Autodesk Inventor part; units mm, degrees
ref_plane "YZ Plane" through (0, 0, 0) normal (1, 0, 0) x (0, 1, 0)
ref_plane "XZ Plane" through (0, 0, 0) normal (0, 1, 0) x (-1, 0, 0)
ref_plane "XY Plane" through (0, 0, 0) normal (0, 0, 1) x (1, 0, 0)
sketch "Sketch1" plane through (0, 0, 0) normal (0, 1, 0) x (-1, 0, 0)
  line L0 (-9.5, 12.5) -> (9.5, 12.5)
  line L1 (12.5, 9.5) -> (12.5, -9.5)
  line L2 (9.5, -12.5) -> (-9.5, -12.5)
  line L3 (-12.5, -9.5) -> (-12.5, 9.5)
  line L4 (-12.5, 12.5) -> (12.5, -12.5) construction
  line L5 (12.5, 12.5) -> (-12.5, -12.5) construction
  line L6 (-10, -10) -> (10, -10) construction
  line L7 (10, -10) -> (10, 10) construction
  line L8 (10, 10) -> (-10, 10) construction
  line L9 (-10, 10) -> (-10, -10) construction
  line L10 (-10, -10) -> (10, 10) construction
  line L11 (10, -10) -> (-10, 10) construction
  circle A0 centre (10, 10) radius 1.2
  circle A1 centre (10, -10) radius 1.2
  circle A2 centre (-10, 10) radius 1.2
  circle A3 centre (-10, -10) radius 1.2
  arc A4 (12.5, 9.5) -> (9.5, 12.5) centre (9.5, 9.5) ccw
  arc A5 (9.5, -12.5) -> (12.5, -9.5) centre (9.5, -9.5) ccw
  arc A6 (-9.5, 12.5) -> (-12.5, 9.5) centre (-9.5, 9.5) ccw
  arc A7 (-12.5, -9.5) -> (-9.5, -12.5) centre (-9.5, -9.5) ccw
  point P0 (0, 0)
  dimension "d0" = 25
  dimension "d1" = 25
  dimension "d2" = 20
  dimension "d3" = 20
  dimension "d4" = 2.4
  dimension "d7" = 20
  dimension "d10" = 20
  dimension "d13" = 3
extrude "Extrusion1" add sketch "Sketch1" along normal blind 3
sketch "Sketch2" plane through (0, 3, 0) normal (0, 1, 0) x (1, 0, 0)
  line L0 (4, -4) -> (-4, -4)
  line L1 (-4, -4) -> (-4, 4)
  line L2 (-4, 4) -> (4, 4)
  line L3 (4, 4) -> (4, -4)
  line L4 (4, -4) -> (-4, 4) construction
  line L5 (-4, -4) -> (4, 4) construction
  point P0 (0, 0)
  dimension "d16" = 8
  dimension "d17" = 8
extrude "Extrusion2" add sketch "Sketch2" along normal blind 3.98
equation "\"d4\" = hole"
equation "\"hole\" = 2.4"
properties part number "camera"
Geometry check sheet. Reference: the model listing, model coordinates, mm. A direction names the side the tool comes from. Round coordinates to 2 decimals unless told otherwise and drop trailing zeros. Order: outer loops, then holes, each group sorted by start corner. A loop starts at its lowest first (then second) coordinate and runs counter-clockwise, first axis right, second up. Notation, with made-up numbers: (50.5, 16.5) -> (80.5, 16.5) arc R32 cw to (80.5, 51.5) -> close; hole circle Ø6 at (78.5, 30). An arc over 180 degrees is marked (long way). Return JSON: item names as keys, results as strings. Group by question number.
Q1. Section check A-A, the plane y = 2. Record the boundary of the cut face in (x, z).
Q2. Tool access check on faces 4 (the flat face through (0, 5, -4)), 5 (the flat face through (4, 5, 0)), 6 (the flat face through (-4, 5, 0)), 7 (the flat face through (0, 5, 4)). Record the directions out of +Z, -Z, +X, -X, +Y, -Y that give a thin tool (end or side, any length) a straight path to the whole face; none if there is none.
Q3. Section check C-C, the plane x = 10. Record the boundary of the cut face in (y, z), plus the area to 3 significant figures.
Q4. Section check D-D, the plane z = 10. Record the boundary of the cut face in (x, y).
Q5. Gauge pin test, flat ends, axial feed: pin 1 (4 mm diameter, centred on x = 6, y = 3.5, fed in from +Z); pin 2 (1 mm diameter, centred on x = 4, z = 8.5, fed in from +Y); pin 3 (1.2 mm diameter, centred on y = 5.5, z = 1.5, fed in from -X); pin 4 (1.5 mm diameter, centred on x = -4.5, y = 5, fed in from +Z). Record the tip position at first contact, or that the pin passes through.
Q6. Section check B-B, the plane z = 1. Record the boundary of the cut face in (x, y).
Q7. Material ranges on probe 1 along Z at (x, y) = (10, 0.95); probe 2 along Y at (x, z) = (9.75, 0.5); probe 3 along Z at (x, y) = (0.25, 6), recorded low to high. Write a range as from..to.
Q8. Release check for a two-part mould opening along Z. For faces 1 (the cylindrical face through (-9.74, 1.48, -8.83)), 2 (the flat face through (0, 1, 12.5)), 3 (the flat face through (12.5, 1, 0)) record: released by +Z, released by -Z, zero draft, split by the parting line, or undercut.
Numbers:
{
 "1": {"outline": "(-12.5, -9.5) arc R3 ccw to (-9.5, -12.5) -> (9.5, -12.5) arc R3 ccw to (12.5, -9.5) -> (12.5, 9.5) arc R3 ccw to (9.5, 12.5) -> (-9.5, 12.5) arc R3 ccw to (-12.5, 9.5) -> close; hole circle Ø2.4 at (-10, -10); hole circle Ø2.4 at (-10, 10); hole circle Ø2.4 at (10, -10); hole circle Ø2.4 at (10, 10)"},
 "2": {"face 4": "-Z, +X, -X, +Y", "face 5": "+Z, -Z, +X, +Y", "face 6": "+Z, -Z, -X, +Y", "face 7": "+Z, +X, -X, +Y"},
 "3": {"outline": "(0, -12.46) -> (3, -12.46) -> (3, -11.2) -> (0, -11.2) -> close; (0, -8.8) -> (3, -8.8) -> (3, 8.8) -> (0, 8.8) -> close; (0, 11.2) -> (3, 11.2) -> (3, 12.46) -> (0, 12.46) -> close", "area": "60.3 mm^2"},
 "4": {"outline": "(-12.46, 0) -> (-11.2, 0) -> (-11.2, 3) -> (-12.46, 3) -> close; (-8.8, 0) -> (8.8, 0) -> (8.8, 3) -> (-8.8, 3) -> close; (11.2, 0) -> (12.46, 0) -> (12.46, 3) -> (11.2, 3) -> close"},
 "5": {"pin 1": "z = 12.5", "pin 2": "y = 3", "pin 3": "x = -4", "pin 4": "z = 4"},
 "6": {"outline": "(-12.5, 0) -> (12.5, 0) -> (12.5, 3) -> (4, 3) -> (4, 6.98) -> (-4, 6.98) -> (-4, 3) -> (-12.5, 3) -> close"},
 "7": {"probe 1": "-12.46..-11.2, -8.8..8.8, 11.2..12.46", "probe 2": "0..3", "probe 3": "-4..4"},
 "8": {"face 1": "undercut", "face 2": "released by +Z", "face 3": "zero draft"}
}
